from build123d import *

# Parameters (mm, degrees)
F1_DEPTH  = 10.95
F2_R      = 1.3
F3_DEPTH  = 1.8
F6_DEPTH  = 5.001
F8_DEPTH  = 13.702198
F9_W      = 11.3
F9_H      = 10.5
F10_DEPTH = 3.647076


with BuildPart() as f1:
    # F0 (on Front) → F1 (new body, symmetric)
    with BuildSketch(Plane.XZ):
        with BuildLine():
            Line((-8.737945, 2.1), (-10.837945, 0))
            Line((-10.837945, 0), (5.062055, 0))
            ThreePointArc((5.062055, 0), (7.540463, 2.827859), (4.412, 4.914007))
            Line((4.412, 4.914007), (-6.037945, 2.1))
            Line((-6.037945, 2.1), (-8.737945, 2.1))
        make_face()
    extrude(amount=F1_DEPTH, both=True)

    # F2 (on face) → F3 (join)
    with BuildSketch(Plane.XZ.offset(10.95)):
        with Locations((5.062055, 2.5)):
            Circle(F2_R)
    extrude(amount=F3_DEPTH)

    # F4: F1 across plane


with BuildPart() as f1_1:
    add(f1.part)
    add(f1.part.mirror(Plane.XZ))

    # F5 (on Top) → F6 (cut, through all)
    with BuildSketch(Plane.XY):
        with BuildLine():
            Line((9.362055, 8.451099), (-2.137945, 8.451099))
            ThreePointArc((-2.137945, 8.451099), (-2.491499, 8.304652), (-2.637945, 7.951099))
            Line((-2.637945, 7.951099), (-2.637945, 7.351099))
            ThreePointArc((-2.637945, 7.351099), (-2.491499, 6.997546), (-2.137945, 6.851099))
            Line((-2.137945, 6.851099), (9.362055, 6.851099))
            Line((9.362055, 6.851099), (9.362055, 8.451099))
        make_face()
        with BuildLine():
            Line((9.362055, -8.451099), (9.362055, -6.851099))
            Line((9.362055, -6.851099), (-2.137945, -6.851099))
            ThreePointArc((-2.137945, -6.851099), (-2.491499, -6.997546), (-2.637945, -7.351099))
            Line((-2.637945, -7.351099), (-2.637945, -7.951099))
            ThreePointArc((-2.637945, -7.951099), (-2.491499, -8.304652), (-2.137945, -8.451099))
            Line((-2.137945, -8.451099), (9.362055, -8.451099))
        make_face()
    extrude(amount=F6_DEPTH, mode=Mode.SUBTRACT)

    # F7 (on face) → F8 (join, through all)
    with BuildSketch(Plane.XZ.offset(6.851099)):
        with BuildLine():
            Line((7.501929, 5.746076), (4.412, 4.914007))
            ThreePointArc((4.412, 4.914007), (7.359868, 3.484913), (6.362029, 0.364569))
            Line((6.362029, 0.364569), (8.776036, 1.014623))
            Line((8.776036, 1.014623), (7.501929, 5.746076))
        make_face()
    extrude(amount=-F8_DEPTH)

    # F9 (on face) → F10 (cut, through all)
    with BuildSketch(Plane.XY.offset(2.1)):
        with Locations((-0.387945, 0)):
            Rectangle(F9_W, F9_H)
    extrude(amount=F10_DEPTH, mode=Mode.SUBTRACT)


solid = f1_1.part
Could you check a few things on this model? Use its own coordinates, in mm. A direction names the side the tool comes from. Give positions to 0.01 mm unless a question says otherwise; leave off trailing zeros. Order: outer loops, then holes, each group sorted by start corner. A loop starts at its lowest first (then second) coordinate and runs counter-clockwise, first axis right, second up. Notation, with made-up numbers: (81.25, 81) - (109.25, 81) arc R19 cw to (109.25, 96) - close; hole circle Ø1 at (85, -15). An arc over 180 degrees is marked (long way). One line per item, written item: value. Start each with the question number.
1. Imagine slicing it at D-D on z = 2.5. List the corners of the cut face in (x, y) for me, plus the area to 3 significant figures.
2. Thinking about a two-plate mould opening in Y: for faces 4 (the face through (5, -12.75, 3)), 5 (the face through (3, 8.451, 2)), 6 (the face through (8.148, -0.096, 3.347)), which applies, +Y half, -Y half, draft (parallel to the pull), parting line (faces both ways), or undercut?
3. Imagine slicing it at C-C on y = -4.75. List the corners of the cut face in (x, z) for me.
4. If I drill on probe 1 along Y at (x, z) = (4.75, 4.6); probe 2 along Y at (x, z) = (1.75, 0.9), over which ranges is the centre line in solid material (lowest first)?
5. Imagine slicing it at A-A on x = 1.25. List the corners of the cut face in (y, z) for me, plus the area to 3 significant figures.
6. For P1, Ø1.7, axis at x = 3, z = 3.5, coming from the +Y side; P2, Ø1.5, axis at x = 2.5, z = 3, coming from the -Y side; P3, Ø11, axis at x = 1, y = -3.5, coming from the +Z side, each with a flat end and sliding along its axis, tell me the tip position at first contact or that it passes through.
7. Imagine slicing it at B-B on z = 4.1. List the corners of the cut face in (x, y) for me, plus the area to 3 significant figures.
8. For faces 1 (the face through (6.3, -11.8, 2.9)), 2 (the face through (2, 5.25, 3)), 3 (the face through (3, -6.851, 2)), which set-ups out of +Z, -Z, +X, -X, +Y, -Y let a thin tool reach every point of the face, with its end or its side?
Values:
1. outline: (-4.55, -10.95) - (3.76, -10.95) - (3.76, -12.75) - (6.36, -12.75) - (6.36, -10.95) - (7.56, -10.95) - (7.56, -8.45) - (-2.14, -8.45) arc R0.5 cw to (-2.64, -7.95) - (-2.64, -7.35) arc R0.5 cw to (-2.14, -6.85) - (8.38, -6.85) - (8.38, 6.85) - (-2.14, 6.85) arc R0.5 cw to (-2.64, 7.35) - (-2.64, 7.95) arc R0.5 cw to (-2.14, 8.45) - (7.56, 8.45) - (7.56, 10.95) - (6.36, 10.95) - (6.36, 12.75) - (3.76, 12.75) - (3.76, 10.95) - (-4.55, 10.95) - (-4.55, 5.25) - (5.26, 5.25) - (5.26, -5.25) - (-4.55, -5.25) - close
1. area: 150 mm²
2. face 4: -Y half
2. face 5: undercut
2. face 6: draft
3. outline: (-10.84, 0) - (5.06, 0) arc R2.5 ccw to (6.36, 0.36) - (8.78, 1.01) - (7.5, 5.75) - (5.26, 5.14) - (5.26, 2.1) - (-8.74, 2.1) - close
4. probe 1: -10.95 to -8.45, -6.85 to -5.25, 5.25 to 6.85, 8.45 to 10.95
4. probe 2: -10.95 to -8.45, -6.85 to 6.85, 8.45 to 10.95
5. outline: (-10.95, 0) - (-8.45, 0) - (-8.45, 4.06) - (-10.95, 4.06) - close; (-6.85, 0) - (6.85, 0) - (6.85, 4.06) - (5.25, 4.06) - (5.25, 2.1) - (-5.25, 2.1) - (-5.25, 4.06) - (-6.85, 4.06) - close; (8.45, 0) - (10.95, 0) - (10.95, 4.06) - (8.45, 4.06) - close
5. area: 55.4 mm²
6. P1: y = 10.95
6. P2: y = -10.95
6. P3: z = 5.48
7. outline: (1.39, -10.95) - (6.98, -10.95) - (6.98, -8.45) - (1.39, -8.45) - close; (1.39, -6.85) - (7.95, -6.85) - (7.95, 6.85) - (1.39, 6.85) - (1.39, 5.25) - (5.26, 5.25) - (5.26, -5.25) - (1.39, -5.25) - close; (1.39, 8.45) - (6.98, 8.45) - (6.98, 10.95) - (1.39, 10.95) - close
7. area: 77.1 mm²
8. face 1: -Y
8. face 2: +Z, -X
8. face 3: +Z, -Z, +X
